Can you work these out from the model? Positions are in its coordinate system, mm. A direction names the side the tool comes from. Give positions to 0.01 mm unless a question says otherwise; leave off trailing zeros. Order: outer loops, then holes, each group sorted by start corner. A loop starts at its lowest first (then second) coordinate and runs counter-clockwise, first axis right, second up. Notation, with made-up numbers: M 54,40.25 L 85,40.25 A20 ccw 85,69.25 Z; hole C -30,83 d2. An arc over 180 degrees is marked long. Use one line per item in the form item = value. Start each with the question number.
1. Will these pins go through, and if not, where does the flat tip stop? P1, Ø1.2, axis at x = 67.5, z = -8, coming from the -Y side; P2, Ø12, axis at x = 49.5, z = -8, coming from the +Y side; P3, Ø2.5, axis at x = 42.5, z = -17, coming from the -Y side.
2. For faces 5 (the face through (28, 40, -17)), 6 (the face through (68.03, 37.75, -3.04)), 7 (the face through (12.981, 25.475, 2.479)), 8 (the face through (28, 35, -16)), 9 (the face through (68, 15, -7)), which set-ups out of +Z, -Z, +X, -X, +Y, -Y let a thin tool reach every point of the face, with its end or its side?
3. I want a section at C-C, the plane y = 4. List the corners of the cut face in (x, z) for me.
4. We'd pull the mould along Z, two halves only. Please class faces 1 (the face through (42, 36, -17)), 2 (the face through (66, 28, -7)), 3 (the face through (-2.1, 20.28, -18.14)), 4 (the face through (69.14, 27.32, 3.1)): +Z half, -Z half, draft (parallel to the pull), parting line (faces both ways), or undercut.
5. I want a section at D-D, the plane z = 0. List the corners of the cut face in (x, y) for me, and give its area (3 significant figures).
6. I want a section at A-A, the plane z = -12. List the corners of the cut face in (x, y) for me, and give its area (3 significant figures).
7. I want a section at B-B, the plane x = 36. List the corners of the cut face in (y, z) for me.
8. I need wall thicknesses on L1, parallel to X at y = 28, z = -15; L2, parallel to Z at x = 0, y = 38; L3, parallel to X at y = 20.5, z = -7.5. Which ranges of each line are inside material? Lowest first, please.
Autodesk Fusion 360 part; units mm, degrees
sketch "Sketch1" plane through (0, 0, 0) normal (0, 1, 0) x (1, 0, 0)
  circle A0 centre (0, 0) radius 1.75
  circle A1 centre (0, 15) radius 1.75
  line L0 (-3, 19) -> (3, 19)
  line L1 (3, 19) -> (3, -4)
  line L2 (3, -4) -> (-3, -4)
  line L3 (-3, -4) -> (-3, 19)
  dimension "d1" = 3.5
  dimension "d2" = 3.5
  dimension "d3" = 15
  dimension "d4" = 4
  dimension "d5" = 4
extrude "Extrude1" add sketch "Sketch1" along normal blind 40 makes body 1
sketch "Sketch2" plane through (0, 40, 0) normal (0, 1, 0) x (-1, 0, 0)
  circle A0 centre (0, -15) radius 1.75
  circle A1 centre (0, 0) radius 1.75
  line L0 (3, 4) -> (-3, 4)
  line L1 (-3, 4) -> (-3, -19)
  line L2 (-3, -19) -> (3, -19)
  line L3 (3, -19) -> (3, 4)
  line L4 (-66, -19) -> (-70, -19)
  line L5 (-70, -19) -> (-70, 4)
  line L6 (-70, 4) -> (-66, 4)
  line L7 (-66, 4) -> (-66, -19)
  dimension "d8" = 4
  dimension "d10" = 70
extrude "Extrude2" add sketch "Sketch2" against normal blind 25 separate body contours L4 L5 L6 L7 makes body 2
sketch "Sketch3" plane through (0, 40, 0) normal (0, 1, 0) x (-1, 0, 0)
  circle A0 centre (0, -15) radius 1.75
  circle A1 centre (0, 0) radius 1.75
  line L0 (3, 4) -> (-3, 4)
  line L1 (-3, 4) -> (-3, -19)
  line L2 (-3, -19) -> (3, -19)
  line L3 (3, -19) -> (3, 4)
  line L4 (-3, -19) -> (-66, -19)
  line L5 (-66, -19) -> (-66, -16)
  line L6 (-66, -16) -> (-3, -16)
  line L7 (-3, -16) -> (-3, -19)
  line L8 (-3, 4) -> (-66, 4)
  line L9 (-66, 4) -> (-66, 1)
  line L10 (-66, 1) -> (-3, 1)
  line L11 (-3, 1) -> (-3, 4)
extrude "Extrude3" add sketch "Sketch3" against normal blind 4 contours L1 L8 L9 L10 L11 | L1 L4 L5 L6 L7 bodies 1 2
fillet "Fillet1" radius 20 2 edges at (66, 36, -17.5) (66, 36, 2.5) on bodies 1
fillet "Fillet2" radius 35 2 edges at (3, 36, -17.5) (3, 36, 2.5) on bodies 1
sketch "Sketch4" plane through (70, 0, 0) normal (1, 0, 0) x (0, 0, -1)
  line L0 (19, 40) -> (-4, 40)
  line L1 (-4, 40) -> (-4, 15)
  line L2 (-4, 15) -> (19, 15)
  line L3 (19, 15) -> (19, 40)
  circle A0 centre (3, 36) radius 1.75
  circle A1 centre (3, 19) radius 1.75
  circle A2 centre (12, 36) radius 1.75
  circle A3 centre (12, 19) radius 1.75
  line L4 (4.75, 19) -> (4.75, 36)
  line L5 (1.25, 36) -> (1.25, 19)
  line L6 (13.75, 36) -> (13.75, 19)
  line L7 (10.25, 19) -> (10.25, 36)
  dimension "d17" = 3.5
  dimension "d18" = 3.5
  dimension "d19" = 3.5
  dimension "d20" = 3.5
  dimension "d21" = 7
  dimension "d22" = 7
  dimension "d23" = 4
  dimension "d24" = 4
extrude "Extrude4" cut sketch "Sketch4" against normal up to surface (4 mm away) contours A0 | A0 A1 L4 L5 | A1 | A2 | A2 A3 L6 L7 | A3 bodies 1
fillet "Fillet3" radius 3 4 edges at (-3, 20, -19) (-3, 20, 4) (70, 27.5, -19) (70, 27.5, 4) on bodies 1
equation "d21 = d22"
equation "d24 = d23"
Check result:
q1.P1 = 15
q1.P2 = through
q1.P3 = 36
q2.face_5 = +Z, -Z, +X, -X, +Y
q2.face_6 = +X
q2.face_7 = +Z, -Z, -Y
q2.face_8 = +Y, -Y
q2.face_9 = +Z, -Z, +X, -Y
q3.outline = M -3,-16 A3 ccw 0,-19 L 3.13,-19 L 3.13,-16 L 3,-16 L 3,1 L 3.13,1 L 3.13,4 L 0,4 A3 ccw -3,1 Z; hole C 0,-15 d3.5; hole C 0,0 d3.5
q4.face_1 = draft
q4.face_2 = undercut
q4.face_3 = -Z half
q4.face_4 = +Z half
q5.outline = M -3,0 L -1.75,0 L -1.75,40 L -3,40 Z; M 1.75,0 L 3,0 L 3,40 L 1.75,40 Z; M 66,15 L 70,15 L 70,40 L 66,40 Z
q5.area = 200 mm2
q6.outline = M -3,0 L 3,0 L 3,40 L -3,40 Z; M 66,15 L 70,15 L 70,17.25 L 66,17.25 Z; M 66,37.75 L 70,37.75 L 70,40 L 66,40 Z
q6.area = 258 mm2
q7.outline = M 35.94,-19 L 40,-19 L 40,-16 L 35.94,-16 Z; M 35.94,1 L 40,1 L 40,4 L 35.94,4 Z
q8.L1 = -3 to -1.75, 1.75 to 3, 66 to 70
q8.L2 = -19 to -16.75, -13.25 to -1.75, 1.75 to 4
q8.L3 = -3 to 3, 66 to 70
